The figure shows three views and two pictorial views of one solid part (mm, origin at its lowest corner). Answer the questions. A direction names the side the tool comes from. Give positions to 0.01 mm unless a question says otherwise; leave off trailing zeros. Loops run counter-clockwise (first coordinate to the right, second up) from the corner with the lowest first, then second, coordinate; pieces in that order, holes last. Notation, with made-up numbers: (-31, 67) - (-27, 67) arc R13 ccw to (-27, 90) - close; hole circle Ø5 at (29.25, -21). An arc over 180 degrees is marked (long way). Use CSV: the item, a comma, the result in double quotes.
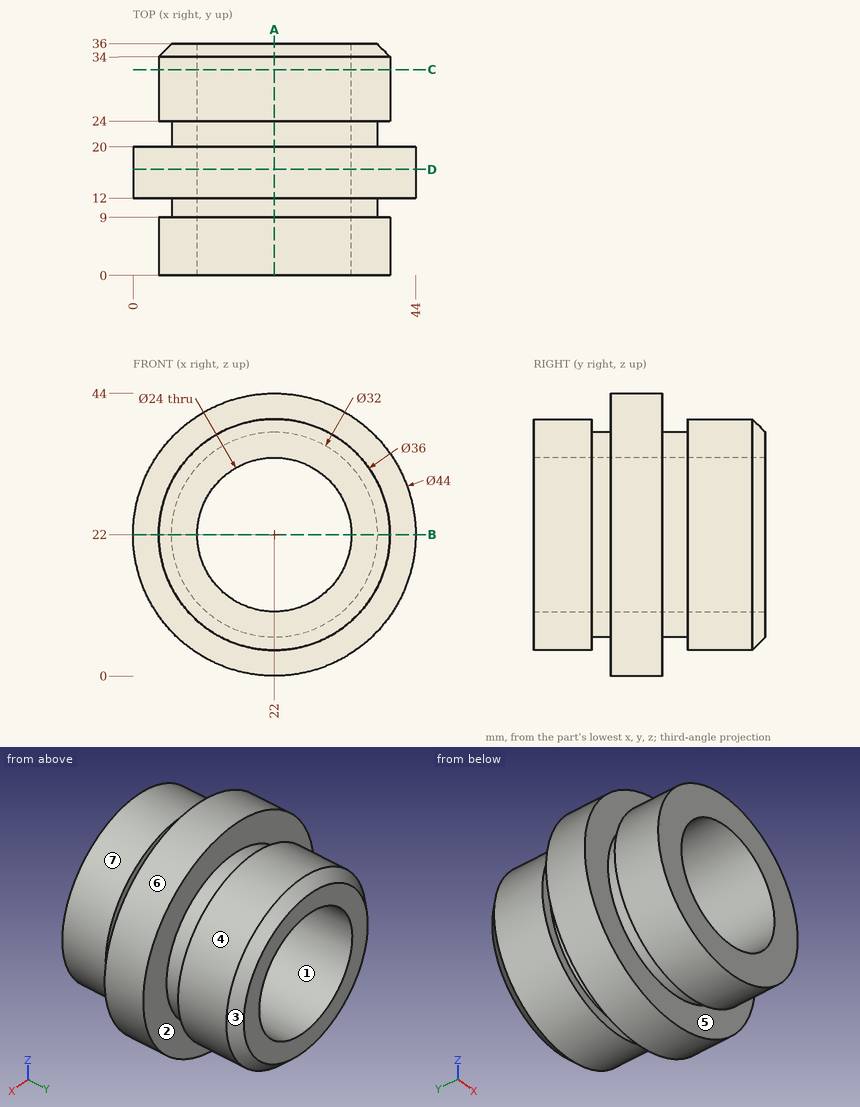
Item 1: Given P1, Ø5, axis at x = 8, y = 15.5, coming from the +Z side (3 decimals); P2, Ø14.5, axis at x = 22, z = 22, coming from the -Y side; P3, Ø10, axis at y = 15, z = 4.5, coming from the -X side; P4, Ø3, axis at y = 11.5, z = 37.5, coming from the +X side, each flat-ended and moving along its own axis, determine where each tip first touches the part or whether it passes through.
Determined:
P1,"stops at z = 40.755"
P2,"passes through"
P3,"stops at x = 3.9"
P4,"stops at x = 38.9"
Item 2: The mould has two halves that part along Z. Classify the marked faces 1, 2 and 3: pulls with the +Z half, pulls with the -Z half, needs draft (parallel to the pull), parting line crosses it, or undercut.
Determined:
face 1,"undercut"
face 2,"needs draft"
face 3,"parting line crosses it"
Item 3: Find the intervals of material crossed by line 1 (X direction, y = 13, z = 22); line 2 (X direction, y = 9.5, z = 22); line 3 (Y direction, x = 6.5, z = 28), in increasing order.
Determined:
line 1,"x = 0 to 10, 34 to 44"
line 2,"x = 6 to 10, 34 to 38"
line 3,"y = 0 to 9, 12 to 20, 24 to 35.38"
Item 4: For the marked faces 4, 5, 6 and 7, determine the directions among +Z, -Z, +X, -X, +Y, -Y from which every point of the face is accessible in a straight line to the end or side of a thin tool.
Determined:
face 4,"+Y"
face 5,"none"
face 6,"+Y, -Y"
face 7,"-Y"
Item 5: A cutting plane is placed at B-B on z = 22. Determine the outline of the cut face in (x, y).
Determined:
outline,"(0, 12) - (6, 12) - (6, 9) - (4, 9) - (4, 0) - (10, 0) - (10, 36) - (6, 36) - (4, 34) - (4, 24) - (6, 24) - (6, 20) - (0, 20) - close; (34, 0) - (40, 0) - (40, 9) - (38, 9) - (38, 12) - (44, 12) - (44, 20) - (38, 20) - (38, 24) - (40, 24) - (40, 34) - (38, 36) - (34, 36) - close"
Item 6: A cutting plane is placed at A-A on x = 22. Determine the outline of the cut face in (y, z), and give its area (3 significant figures).
Determined:
outline,"(0, 4) - (9, 4) - (9, 6) - (12, 6) - (12, 0) - (20, 0) - (20, 6) - (24, 6) - (24, 4) - (34, 4) - (36, 6) - (36, 10) - (0, 10) - close; (0, 34) - (36, 34) - (36, 38) - (34, 40) - (24, 40) - (24, 38) - (20, 38) - (20, 44) - (12, 44) - (12, 38) - (9, 38) - (9, 40) - (0, 40) - close"
area,"464 mm²"
Item 7: A cutting plane is placed at D-D on y = 16.5. Determine the outline of the cut face in (x, z).
Determined:
outline,"circle Ø44 at (22, 22); hole circle Ø24 at (22, 22)"
Item 8: A cutting plane is placed at C-C on y = 32. Determine the outline of the cut face in (x, z).
Determined:
outline,"circle Ø36 at (22, 22); hole circle Ø24 at (22, 22)"
